Design review of the part built by this model. Coordinates are the model's own, in mm. Face numbers are marked on the shaded views. Round coordinates to 2 decimals unless told otherwise and drop trailing zeros. Loops run counter-clockwise (first coordinate to the right, second up) from the corner with the lowest first, then second, coordinate; pieces in that order, holes last. Notation, with made-up numbers: (48.25, -21) -> (92.25, -21) arc R20 ccw to (92.25, 11) -> close; hole circle Ø5 at (76, 46). An arc over 180 degrees is marked (long way). Use a Markdown table: item, result. Add a question column.
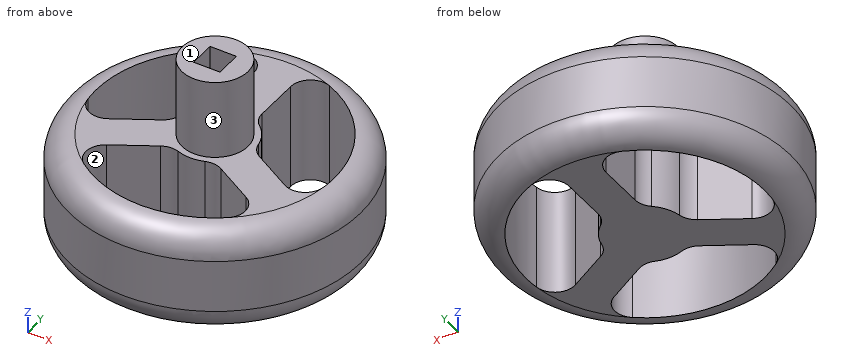
from build123d import *

# Parameters (mm, degrees)
SKETCH1_R           = 27.94
BOSS_EXTRUDE1_DEPTH = 20.32
SKETCH2_R           = 6.35
BOSS_EXTRUDE2_DEPTH = 20.32
BOSS_EXTRUDE3_START = 20.32
SKETCH3_R           = 27.94
BOSS_EXTRUDE3_DEPTH = 20.32
FILLET1_R           = 5.08
FILLET2_R           = 5.08
FILLET3_R           = 5.08
FILLET4_R           = 5.08
CUT_EXTRUDE1_DEPTH  = 73.645776241
SKETCH6_R           = 27.94
CUT_EXTRUDE2_DEPTH  = 57.682420605
SKETCH7_R           = 6.35
CUT_EXTRUDE3_DEPTH  = 5.08
SKETCH8_W           = 5.08
SKETCH8_H           = 5.08
CUT_EXTRUDE4_DEPTH  = 12.7


with BuildPart() as part:
    # Sketch1 → Boss-Extrude1 (new body)
    with BuildSketch(Plane.XY):
        Circle(SKETCH1_R)
    extrude(amount=BOSS_EXTRUDE1_DEPTH)

    # Sketch2 → Boss-Extrude2 (add)
    with BuildSketch(Plane(origin=(0, 0, 0), x_dir=(-1, 0, 0), z_dir=(0, 0, -1))):
        with Locations(Location((0, 0, 0), (0, 0, 180))):
            Circle(SKETCH2_R)
    extrude(amount=BOSS_EXTRUDE2_DEPTH)

    # Sketch3 → Boss-Extrude3 (add)
    with BuildSketch(Plane(origin=(0, 0, -20.32), x_dir=(-1, 0, 0), z_dir=(0, 0, -1)).offset(BOSS_EXTRUDE3_START)):
        with Locations(Location((0, 0, 0), (0, 0, 180))):
            Circle(SKETCH3_R)
    extrude(amount=-BOSS_EXTRUDE3_DEPTH)

    # Fillet1
    fillet1_edges = [part.edges().sort_by_distance(p)[0] for p in [
        (-27.94, 0, 20.32),
    ]]
    fillet(fillet1_edges, radius=FILLET1_R)

    # Fillet2
    fillet2_edges = [part.edges().sort_by_distance(p)[0] for p in [
        (-27.94, 0, 0),
    ]]
    fillet(fillet2_edges, radius=FILLET2_R)

    # Fillet3
    fillet3_edges = [part.edges().sort_by_distance(p)[0] for p in [
        (-27.94, 0, -20.32),
    ]]
    fillet(fillet3_edges, radius=FILLET3_R)

    # Fillet4
    fillet4_edges = [part.edges().sort_by_distance(p)[0] for p in [
        (-27.94, 0, -40.64),
    ]]
    fillet(fillet4_edges, radius=FILLET4_R)

    # Sketch4 → Cut-Extrude1 (cut, through all)
    with BuildSketch(Plane(origin=(0, 0, -40.64), x_dir=(-1, 0, 0), z_dir=(0, 0, -1))):
        with BuildLine():
            Line((-3.556, 8.739962471), (-3.556, 17.568282329))
            ThreePointArc((-3.556, 17.568282329), (-5.256117539, 20.740741312), (-8.8392, 21.081938795))
            ThreePointArc((-8.8392, 21.081938795), (-19.797340731, 11.43), (-22.677094558, -2.885997648))
            ThreePointArc((-22.677094558, -2.885997648), (-20.590067639, -5.818439342), (-16.992578798, -5.704554829))
            Line((-16.992578798, -5.704554829), (-9.347029528, -1.2903949))
            ThreePointArc((-9.347029528, -1.2903949), (-8.133427478, -0.179541209), (-7.501353019, 1.339441259))
            ThreePointArc((-7.501353019, 1.339441259), (-6.599113577, 3.81), (-4.910666667, 5.826641648))
            ThreePointArc((-4.910666667, 5.826641648), (-3.911226491, 7.13352542), (-3.556, 8.739962471))
        make_face()
        with BuildLine():
            Line((3.556, 8.739962471), (3.556, 17.568282329))
            ThreePointArc((3.556, 17.568282329), (5.256117539, 20.740741312), (8.8392, 21.081938795))
            ThreePointArc((8.8392, 21.081938795), (19.797340731, 11.43), (22.677094558, -2.885997648))
            ThreePointArc((22.677094558, -2.885997648), (20.590067639, -5.818439342), (16.992578798, -5.704554829))
            Line((16.992578798, -5.704554829), (9.347029528, -1.2903949))
            ThreePointArc((9.347029528, -1.2903949), (8.133427478, -0.179541209), (7.501353019, 1.339441259))
            ThreePointArc((7.501353019, 1.339441259), (6.599113577, 3.81), (4.910666667, 5.826641648))
            ThreePointArc((4.910666667, 5.826641648), (3.911226491, 7.13352542), (3.556, 8.739962471))
        make_face()
        with BuildLine():
            Line((5.791029528, -7.449567572), (13.436578798, -11.8637275))
            ThreePointArc((13.436578798, -11.8637275), (15.3339501, -14.92230197), (13.837894558, -18.195941147))
            ThreePointArc((13.837894558, -18.195941147), (0, -22.86), (-13.837894558, -18.195941147))
            ThreePointArc((-13.837894558, -18.195941147), (-15.3339501, -14.92230197), (-13.436578798, -11.8637275))
            Line((-13.436578798, -11.8637275), (-5.791029528, -7.449567572))
            ThreePointArc((-5.791029528, -7.449567572), (-4.222200987, -6.953984211), (-2.590686352, -7.166082907))
            ThreePointArc((-2.590686352, -7.166082907), (0, -7.62), (2.590686352, -7.166082907))
            ThreePointArc((2.590686352, -7.166082907), (4.222200987, -6.953984211), (5.791029528, -7.449567572))
        make_face()
    extrude(amount=-CUT_EXTRUDE1_DEPTH, mode=Mode.SUBTRACT)

    # Sketch6 → Cut-Extrude2 (cut, through all)
    with BuildSketch(Plane(origin=(0, 0, 0), x_dir=(-1, 0, 0), z_dir=(0, 0, -1))):
        Circle(SKETCH6_R)
    extrude(amount=-CUT_EXTRUDE2_DEPTH, mode=Mode.SUBTRACT)

    # Sketch7 → Cut-Extrude3 (cut)
    with BuildSketch(Plane.XY):
        Circle(SKETCH7_R)
    extrude(amount=-CUT_EXTRUDE3_DEPTH, mode=Mode.SUBTRACT)

    # Sketch8 → Cut-Extrude4 (cut)
    with BuildSketch(Plane.XY.offset(-5.08)):
        Rectangle(SKETCH8_W, SKETCH8_H)
    extrude(amount=-CUT_EXTRUDE4_DEPTH, mode=Mode.SUBTRACT)


solid = part.part
1. To check wall thickness, follow probe 1 along Y at (x, z) = (0.5, -31); probe 2 along Z at (x, y) = (-18, -13); probe 3 along X at (y, z) = (20, -31.5). State the ranges of each line that lie inside material, in increasing order. Write a range as from..to.
2. Consider section D-D on x = -11. Give the number of separate pieces and of enclosed holes in the cut face, plus the area to 3 significant figures.
3. Mouldability with a two-part tool opening along X and no side actions: class the marked faces 1, 2 and 3 as +X half, -X half, draft (parallel to the pull), parting line (faces both ways), or undercut.
4. Insertion check: P1, Ø3, axis at x = 4, z = -26, coming from the -Y side; P2, Ø1.5, axis at y = 1, z = -9, coming from the +X side; P3, Ø2.5, axis at y = 12.5, z = -28, coming from the -X side (3 decimals). Each pin has a flat end and moves straight along its axis. Give the tip position at first contact, or say it passes through.
5. Consider section C-C on y = 0. State the section outline as (x, z) points, plus the area to 3 significant figures.
6. Consider section A-A on z = -31. State the section outline as (x, y) points (3 decimals), plus the area to 3 significant figures.
7. Consider section B-B on x = 0. State the section outline as (y, z) points.
Verdict:
| question | item | result |
|---|---|---|
| 1 | probe 1 | y = -27.94..-22.85, -7.6..27.94 |
| 1 | probe 2 | z = -40.64..-20.32 |
| 1 | probe 3 | x = -19.51..-11.07, -4.43..4.43, 11.07..19.51 |
| 2 | separate pieces | 3 |
| 2 | enclosed holes | 0 |
| 2 | area | 372 mm² |
| 3 | face 1 | draft |
| 3 | face 2 | undercut |
| 3 | face 3 | parting line |
| 4 | P1 | stops at y = -27.83 |
| 4 | P2 | stops at x = 6.35 |
| 4 | P3 | stops at x = -25.575 |
| 5 | outline | (-27.94, -35.56) arc R5.08 ccw to (-22.86, -40.64) -> (-22.86, -20.32) arc R5.08 ccw to (-27.94, -25.4) -> close; (-8.01, -40.64) -> (8.01, -40.64) -> (8.01, -20.32) -> (6.35, -20.32) -> (6.35, -5.08) -> (2.54, -5.08) -> (2.54, -17.78) -> (-2.54, -17.78) -> (-2.54, -5.08) -> (-6.35, -5.08) -> (-6.35, -20.32) -> (-8.01, -20.32) -> close; (22.86, -40.64) arc R5.08 ccw to (27.94, -35.56) -> (27.94, -25.4) arc R5.08 ccw to (22.86, -20.32) -> close |
| 5 | area | 639 mm² |
| 6 | outline | circle Ø55.88 at (0, 0); hole (-22.677, -2.886) arc R3.81 ccw to (-16.993, -5.705) -> (-9.347, -1.29) arc R3.81 ccw to (-7.501, 1.339) arc R7.62 cw to (-4.911, 5.827) arc R3.81 ccw to (-3.556, 8.74) -> (-3.556, 17.568) arc R3.81 ccw to (-8.839, 21.082) arc R22.86 ccw to start; hole (-13.838, -18.196) arc R22.86 ccw to (13.838, -18.196) arc R3.81 ccw to (13.437, -11.864) -> (5.791, -7.45) arc R3.81 ccw to (2.591, -7.166) arc R7.62 cw to (-2.591, -7.166) arc R3.81 ccw to (-5.791, -7.45) -> (-13.437, -11.864) arc R3.81 ccw to start; hole (3.556, 8.74) arc R3.81 ccw to (4.911, 5.827) arc R7.62 cw to (7.501, 1.339) arc R3.81 ccw to (9.347, -1.29) -> (16.993, -5.705) arc R3.81 ccw to (22.677, -2.886) arc R22.86 ccw to (8.839, 21.082) arc R3.81 ccw to (3.556, 17.568) -> close |
| 6 | area | 1,360 mm² |
| 7 | outline | (-27.94, -35.56) arc R5.08 ccw to (-22.86, -40.64) -> (-22.86, -20.32) arc R5.08 ccw to (-27.94, -25.4) -> close; (-7.62, -40.64) -> (22.86, -40.64) arc R5.08 ccw to (27.94, -35.56) -> (27.94, -25.4) arc R5.08 ccw to (22.86, -20.32) -> (6.35, -20.32) -> (6.35, -5.08) -> (2.54, -5.08) -> (2.54, -17.78) -> (-2.54, -17.78) -> (-2.54, -5.08) -> (-6.35, -5.08) -> (-6.35, -20.32) -> (-7.62, -20.32) -> close |
